from build123d import *

# Parameters (mm, degrees)
SKETCH_1_W                       = 4
SKETCH_1_H                       = 4
EXTRUDE_1_DEPTH                  = 290
FILLET_1_R                       = 1
FILLET_2_R                       = 2
FILLET_3_R                       = 0.5
PATTERN_CIRCULAR_1_COUNT         = 4
FILLET_1_OF_PATTERN_CIRCULAR_1_R = 1
FILLET_2_OF_PATTERN_CIRCULAR_1_R = 2
FILLET_3_OF_PATTERN_CIRCULAR_1_R = 0.5
SKETCH_2_R                       = 3.4
CUT_EXTRUDE_1_DEPTH              = 291
SKETCH_3_R                       = 3.05
CUT_EXTRUDE_2_DEPTH              = 10


with BuildPart() as part:
    # 草图1 → 凸台-拉伸1 (new body)
    with BuildSketch(Plane.XY):
        Polygon((5.7, 0), (5.7, 4.427207794), (9.672792206, 8.4), (13.2, 8.4), (13.2, 4.1), (14.1, 4.1), (14.1, 5.1), (15, 5.1), (15, 15), (5.1, 15), (5.1, 14.1), (4.1, 14.1), (4.1, 13.2), (8.4, 13.2), (8.4, 9.672792206), (4.427207794, 5.7), (0, 5.7), (0, 0), align=None)
        with Locations((11.7, 11.7)):
            Rectangle(SKETCH_1_W, SKETCH_1_H, mode=Mode.SUBTRACT)
    extrude_1 = extrude(amount=EXTRUDE_1_DEPTH)

    # 圆角1
    fillet_1_edges = [part.edges().sort_by_distance(p)[0] for p in [
        (13.7, 9.7, 145),
        (13.7, 13.7, 145),
        (9.7, 13.7, 145),
        (9.7, 9.7, 145),
    ]]
    fillet(fillet_1_edges, radius=FILLET_1_R)

    # 圆角2
    fillet_2_edges = [part.edges().sort_by_distance(p)[0] for p in [
        (15, 15, 145),
    ]]
    fillet(fillet_2_edges, radius=FILLET_2_R)

    # 圆角3
    fillet_3_edges = [part.edges().sort_by_distance(p)[0] for p in [
        (4.427207794, 5.7, 145),
        (8.4, 9.672792206, 145),
        (8.4, 13.2, 145),
        (13.2, 8.4, 145),
        (9.672792206, 8.4, 145),
        (5.7, 4.427207794, 145),
    ]]
    fillet(fillet_3_edges, radius=FILLET_3_R)

    # 阵列(圆周)1: 凸台-拉伸1 ×4 about axis
    pattern_circular_1_axis = Axis((0, 0, 0), (0, 0, 1))
    for i in range(1, PATTERN_CIRCULAR_1_COUNT):
        add(extrude_1.rotate(pattern_circular_1_axis, i * 360 / PATTERN_CIRCULAR_1_COUNT))

    # 圆角1 of 阵列(圆周)1
    fillet_1_of_pattern_circular_1_edges = [part.edges().sort_by_distance(p)[0] for p in [
        (-9.7, 13.7, 145),
        (-13.7, 13.7, 145),
        (-13.7, 9.7, 145),
        (-9.7, 9.7, 145),
        (-13.7, -9.7, 145),
        (-13.7, -13.7, 145),
        (-9.7, -13.7, 145),
        (-9.7, -9.7, 145),
        (9.7, -13.7, 145),
        (13.7, -13.7, 145),
        (13.7, -9.7, 145),
        (9.7, -9.7, 145),
    ]]
    fillet(fillet_1_of_pattern_circular_1_edges, radius=FILLET_1_OF_PATTERN_CIRCULAR_1_R)

    # 圆角2 of 阵列(圆周)1
    fillet_2_of_pattern_circular_1_edges = [part.edges().sort_by_distance(p)[0] for p in [
        (-15, 15, 145),
        (-15, -15, 145),
        (15, -15, 145),
    ]]
    fillet(fillet_2_of_pattern_circular_1_edges, radius=FILLET_2_OF_PATTERN_CIRCULAR_1_R)

    # 圆角3 of 阵列(圆周)1
    fillet_3_of_pattern_circular_1_edges = [part.edges().sort_by_distance(p)[0] for p in [
        (-5.7, 4.427207794, 145),
        (-9.672792206, 8.4, 145),
        (-13.2, 8.4, 145),
        (-8.4, 13.2, 145),
        (-8.4, 9.672792206, 145),
        (-4.427207794, 5.7, 145),
        (-4.427207794, -5.7, 145),
        (-8.4, -9.672792206, 145),
        (-8.4, -13.2, 145),
        (-13.2, -8.4, 145),
        (-9.672792206, -8.4, 145),
        (-5.7, -4.427207794, 145),
        (5.7, -4.427207794, 145),
        (9.672792206, -8.4, 145),
        (13.2, -8.4, 145),
        (8.4, -13.2, 145),
        (8.4, -9.672792206, 145),
        (4.427207794, -5.7, 145),
    ]]
    fillet(fillet_3_of_pattern_circular_1_edges, radius=FILLET_3_OF_PATTERN_CIRCULAR_1_R)

    # 草图2 → 切除-拉伸1 (cut, through all)
    with BuildSketch(Plane.XY.offset(290)):
        Circle(SKETCH_2_R)
    extrude(amount=-CUT_EXTRUDE_1_DEPTH, mode=Mode.SUBTRACT)

    # 草图3 → 切除-拉伸2 (cut, symmetric)
    with BuildSketch(Plane(origin=(0, 0, 0), x_dir=(0, 0, -1), z_dir=(1, 0, 0))):
        with Locations((-145, 0)):
            Circle(SKETCH_3_R)
    extrude(amount=CUT_EXTRUDE_2_DEPTH, both=True, mode=Mode.SUBTRACT)


solid = part.part
Work out the finished part from the listing and answer in its coordinate system (mm). Round coordinates to 2 decimals unless told otherwise and drop trailing zeros. Answer as CSV lines item,"result". Start each with the question number.
(1) The mould has two halves that part along X. Classify faces 1 (the flat face through (15, -9, 143)), 2 (the flat face through (9, -15, 143)), 3 (the flat face through (0, 5.7, 143)): +X half, -X half, draft (parallel to the pull), parting line (faces both ways), or undercut.
(2) Find the intervals of material crossed by probe 1 along X at (y, z) = (-11.5, 94.5); probe 2 along Y at (x, z) = (0, 85), in increasing order.
(3) Each of these flat-tipped pins is pushed along its axis until it touches: pin 1 (10 mm diameter, centred on y = 2.5, z = 151, fed in from -X); pin 2 (0.5 mm diameter, centred on y = -14.5, z = 173, fed in from -X); pin 3 (0.7 mm diameter, centred on x = -14.5, z = 159, fed in from +Y); pin 4 (0.5 mm diameter, centred on x = 4.5, z = 213.5, fed in from +Y). Where does it stop, or does it pass through?
(4) The part is cut by section A-A, the plane z = 81.5. Give the number of separate pieces and of enclosed holes in the cut face, then the cut area to 3 significant figures.
Output values:
1,face 1,"+X half"
1,face 2,"draft"
1,face 3,"undercut"
2,probe 1,"x = -15 to -13.7, -9.7 to -8.4, 8.4 to 9.7, 13.7 to 15"
2,probe 2,"y = -5.7 to -3.4, 3.4 to 5.7"
3,pin 1,"stops at x = -15"
3,pin 2,"stops at x = -14.56"
3,pin 3,"stops at y = 14.64"
3,pin 4,"stops at y = 14.1"
4,separate pieces,"1"
4,enclosed holes,"5"
4,area,"293 mm²"
